Check sheet for the drawn part. Datum: minimum x, y, z corner. Units: mm. A direction names the side the tool comes from. Coordinates: 2 decimals unless noted, no trailing zeros. Order: outer loops, then holes, each group sorted by start corner. A loop starts at its lowest first (then second) coordinate and runs counter-clockwise, first axis right, second up. Notation, with made-up numbers: (-26, 6.5) - (-1, 6.5) arc R28 ccw to (-1, 26.5) - close; hole circle Ø1 at (18.5, 32.25). An arc over 180 degrees is marked (long way). Return JSON: item names as keys, results as strings. Group by question number.
Item 1: Scan lines: probe 1 along X at (y, z) = (21, 15); probe 2 along Z at (x, y) = (101, 34); probe 3 along X at (y, z) = (12, 29.5). Record each from-to range of solid material in increasing order.
Item 2: Gauge pin test, flat ends, axial feed: pin 1 (3 mm diameter, centred on x = 111.5, z = 49, fed in from -Y); pin 2 (10 mm diameter, centred on y = 19.5, z = 46.5, fed in from +X); pin 3 (7.5 mm diameter, centred on y = 24.5, z = 15, fed in from +X); pin 4 (23 mm diameter, centred on x = 101.6, z = 28.575, fed in from -Y). Record the tip position at first contact, or that the pin passes through.
Item 3: Section check C-C on z = 21. Enter the section's corners in (x, y), then the cut area to 3 significant figures.
Item 4: Tool access check on the marked faces 4, 5 and 6. Record the directions out of +Z, -Z, +X, -X, +Y, -Y that give a thin tool (end or side, any length) a straight path to the whole face; none if there is none.
Item 5: Draft check along X on the marked faces 1, 2 and 3. Enter one of: pulls with the +X half, pulls with the -X half, needs draft (parallel to the pull), parting line crosses it, or undercut.
Item 6: Section check B-B on y = 24. Enter the section's corners in (x, z), then the cut area to 3 significant figures.
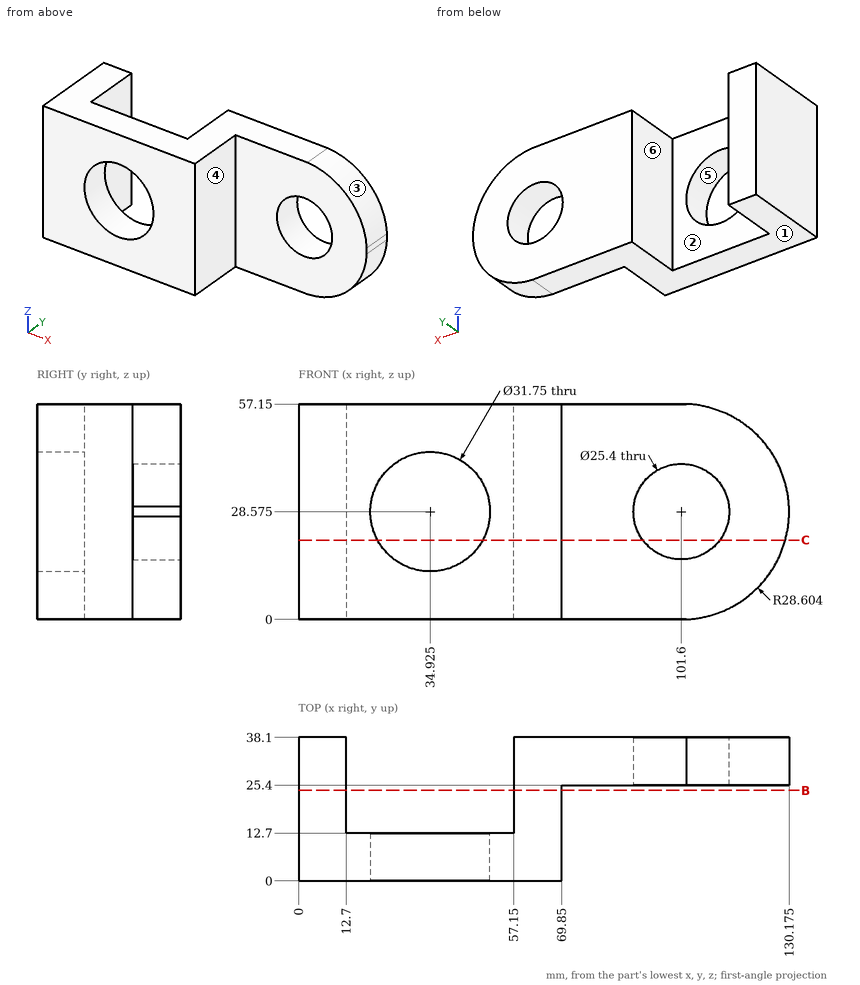
Computed:
{
 "1": {"probe 1": "x = 0 to 12.7, 57.15 to 69.85", "probe 2": "z = 0 to 15.89, 41.26 to 57.15", "probe 3": "x = 0 to 19.08, 50.77 to 69.85"},
 "2": {"pin 1": "stops at y = 25.4", "pin 2": "stops at x = 69.85", "pin 3": "stops at x = 128.42", "pin 4": "passes through"},
 "3": {"outline": "(0, 0) - (20.97, 0) - (20.97, 12.7) - (12.7, 12.7) - (12.7, 38.1) - (0, 38.1) - close; (48.88, 0) - (69.85, 0) - (69.85, 25.4) - (91.41, 25.4) - (91.41, 38.1) - (57.15, 38.1) - (57.15, 12.7) - (48.88, 12.7) - close; (111.79, 25.4) - (129.18, 25.4) - (129.18, 38.1) - (111.79, 38.1) - close", "area": "1,670 mm²"},
 "4": {"face 4": "+Z, -Z, +X, -Y", "face 5": "+Y, -Y", "face 6": "+Z, -Z, +Y"},
 "5": {"face 1": "needs draft", "face 2": "undercut", "face 3": "pulls with the +X half"},
 "6": {"outline": "(0, 0) - (12.7, 0) - (12.7, 57.15) - (0, 57.15) - close; (57.15, 0) - (69.85, 0) - (69.85, 57.15) - (57.15, 57.15) - close", "area": "1,450 mm²"}
}
